Could you check a few things on this model? Use its own coordinates, in mm. A direction names the side the tool comes from. Coordinates: 2 decimals unless noted, no trailing zeros. Write each loop counter-clockwise with the first axis right and the second up, starting at its lowest first coordinate (ties: lowest second). Pieces come first, ordered by that corner, then holes.
```python
from build123d import *

# Parameters (mm, degrees)
SKETCH1_W           = 23.905693463
SKETCH1_H           = 28.387398435
BOSS_EXTRUDE1_DEPTH = 30
SKETCH3_W           = 21.980836904
SKETCH3_H           = 42
BOSS_EXTRUDE2_DEPTH = 23.905693
SKETCH2_R           = 4.775946378
CUT_EXTRUDE1_DEPTH  = 54.417670701


with BuildPart() as part:
    # Sketch1 → Boss-Extrude1 (new body)
    with BuildSketch(Plane.XY):
        with Locations((-0.452846732, 0.006300783)):
            Rectangle(SKETCH1_W, SKETCH1_H)
    extrude(amount=BOSS_EXTRUDE1_DEPTH)

    # Sketch3 → Boss-Extrude2 (add, through all)
    with BuildSketch(Plane(origin=(11.5, 0, 0), x_dir=(0, 0, -1), z_dir=(1, 0, 0))):
        with Locations((-19.596283116, 0.006300783)):
            Rectangle(SKETCH3_W, SKETCH3_H)
    extrude(amount=-BOSS_EXTRUDE2_DEPTH)

    # Sketch2 → Cut-Extrude1 (cut, through all)
    with BuildSketch(Plane(origin=(0, 21.006300783, 0), x_dir=(1, 0, 0), z_dir=(0, 1, 0))):
        with Locations(Location((0, -20.454249212, 0), (0, 0, 270))):
            Circle(SKETCH2_R)
    extrude(amount=-CUT_EXTRUDE1_DEPTH, mode=Mode.SUBTRACT)


solid = part.part
```
1. I want a section at A-A on x = 0. Please give me the cut outline in (y, z), plus the area to 3 significant figures.
Verdict:
outline: (-20.99, 8.61) - (-14.19, 8.61) - (-14.19, 0) - (14.2, 0) - (14.2, 8.61) - (21.01, 8.61) - (21.01, 15.68) - (-20.99, 15.68) - close; (-20.99, 25.23) - (21.01, 25.23) - (21.01, 30.59) - (-20.99, 30.59) - close
area: 766 mm2
2. On a 3-axis mill with a long thin cutter (end or side, diameter ignored), from which of +Z, -Z, +X, -X, +Y, -Y can I reach the whole of each face in a straight line? I mean faces 4 (the face through (-1, 0, 0)), 5 (the face through (-1, 14.2, 4)), 6 (the face through (-1, -14.187, 4)). Say none if no direction works.
Verdict:
face 4: -Z, +X, -X, +Y, -Y
face 5: -Z, +X, -X, +Y
face 6: -Z, +X, -X, -Y
3. If we mould it in two halves opening along Z, with no side actions, what happens to faces 1 (the face through (0, -20.994, 15)), 2 (the face through (0.21, 0.3, 15.683)), 3 (the face through (0, -18, 8.606))? For each: pulls with the +Z half, pulls with the -Z half, needs draft (parallel to the pull), parting line crosses it, or undercut.
Verdict:
face 1: needs draft
face 2: undercut
face 3: pulls with the -Z half
4. I want a section at B-B on z = 21.5. Please give me the cut outline in (x, y), plus the area to 3 significant figures.
Verdict:
outline: (-12.41, -20.99) - (-4.66, -20.99) - (-4.66, 21.01) - (-12.41, 21.01) - close; (4.66, -20.99) - (11.5, -20.99) - (11.5, 21.01) - (4.66, 21.01) - close
area: 613 mm2
5. I want a section at C-C on y = 11. Please give me the cut outline in (x, z), plus the area to 3 significant figures.
Verdict:
outline: (-12.41, 0) - (11.5, 0) - (11.5, 30.59) - (-12.41, 30.59) - close; hole circle Ø9.55 at (0, 20.45)
area: 660 mm2
6. I want a section at D-D on x = -9.5. Please give me the cut outline in (y, z), plus the area to 3 significant figures.
Verdict:
outline: (-20.99, 8.61) - (-14.19, 8.61) - (-14.19, 0) - (14.2, 0) - (14.2, 8.61) - (21.01, 8.61) - (21.01, 30.59) - (-20.99, 30.59) - close
area: 1,170 mm2
7. Please list where these lines run through material, in increasing order: line 1 along X through (y, z) = (14, 21.5); line 2 along Y through (x, z) = (-1.5, 5); line 3 along X through (y, z) = (-15, 23.5).
Verdict:
line 1: x = -12.41 to -4.66, 4.66 to 11.5
line 2: y = -14.19 to 14.2
line 3: x = -12.41 to -3.68, 3.68 to 11.5
8. For pin 1 (3.5 mm diameter, centred on x = -4, y = 17.5, fed in from -Z), with a flat end and sliding along its axis, tell me the tip position at first contact or that it passes through.
Verdict:
pin 1: stops at z = 8.61
